Part model, mm, in its own coordinate system. Round coordinates to 2 decimals unless told otherwise and drop trailing zeros. Loops run counter-clockwise (first coordinate to the right, second up) from the corner with the lowest first, then second, coordinate; pieces in that order, holes last.
(1) Flat gauge pin, fed straight in: pin 1 (5 mm diameter, centred on x = 190, z = 155, fed in from +Y). Where does the tip first touch, or does it go through?
(2) Probe probe 1 along X at (y, z) = (-5.75, 204.5); probe 2 along X at (y, z) = (-4, 337.4); probe 3 along X at (y, z) = (-3.75, 125). List the from-to ranges inside material, lowest first.
(3) Cut at B-B on z = 61. List the corners of the cut face in (x, y), then the cut area to 3 significant figures.
(4) Cut at A-A on z = 125. List the corners of the cut face in (x, y), then the cut area to 3 significant figures.
(5) Cut at C-C on y = -8.25. Count the separate pieces of the cut face and the enclosed holes in it, then the cut area to 3 significant figures.
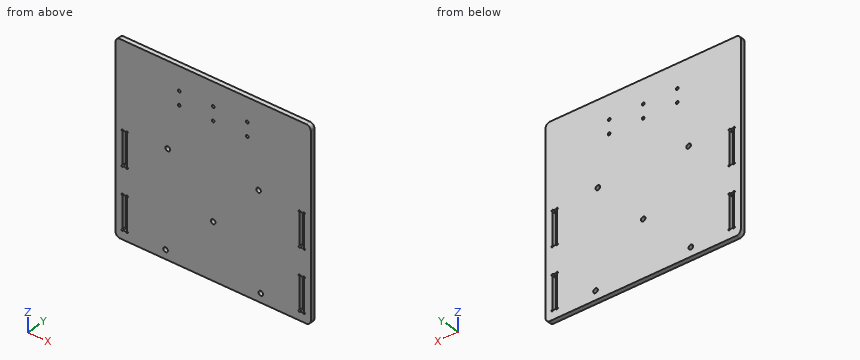
from build123d import *

# Parameters (mm, degrees)
F0_R     = 5.1
F0_R_2   = 3
F1_DEPTH = 10
F2_R     = 10


with BuildPart() as f1:
    # F0 (on Front) → F1 (new body)
    with BuildSketch(Plane.XZ):
        Polygon((-215, 0), (0, 0), (215, 0), (215, 420), (0, 420), (-215, 420), align=None)
        with BuildLine():
            ThreePointArc((-198, 20), (-201.414214, 18.585786), (-200, 22))
            Line((-200, 22), (-200, 93))
            ThreePointArc((-200, 93), (-201.414214, 96.414214), (-198, 95))
            Line((-198, 95), (-192, 95))
            ThreePointArc((-192, 95), (-188.585786, 96.414214), (-190, 93))
            Line((-190, 93), (-190, 22))
            ThreePointArc((-190, 22), (-188.585786, 18.585786), (-192, 20))
            Line((-192, 20), (-198, 20))
        make_face(mode=Mode.SUBTRACT)
        with Locations((-105, 20)):
            Circle(F0_R, mode=Mode.SUBTRACT)
        with BuildLine():
            Line((-192, 155), (-198, 155))
            ThreePointArc((-198, 155), (-201.414214, 153.585786), (-200, 157))
            Line((-200, 157), (-200, 228))
            ThreePointArc((-200, 228), (-201.414214, 231.414214), (-198, 230))
            Line((-198, 230), (-192, 230))
            ThreePointArc((-192, 230), (-188.585786, 231.414214), (-190, 228))
            Line((-190, 228), (-190, 157))
            ThreePointArc((-190, 157), (-188.585786, 153.585786), (-192, 155))
        make_face(mode=Mode.SUBTRACT)
        with Locations((105, 20)):
            Circle(F0_R, mode=Mode.SUBTRACT)
        with BuildLine():
            ThreePointArc((190, 93), (188.585786, 96.414214), (192, 95))
            Line((192, 95), (198, 95))
            ThreePointArc((198, 95), (201.414214, 96.414214), (200, 93))
            Line((200, 93), (200, 22))
            ThreePointArc((200, 22), (201.414214, 18.585786), (198, 20))
            Line((198, 20), (192, 20))
            ThreePointArc((192, 20), (188.585786, 18.585786), (190, 22))
            Line((190, 22), (190, 93))
        make_face(mode=Mode.SUBTRACT)
        with BuildLine():
            ThreePointArc((0, 119.9), (-5.1, 125), (0, 130.1))
            ThreePointArc((0, 130.1), (5.1, 125), (0, 119.9))
        make_face(mode=Mode.SUBTRACT)
        with BuildLine():
            Line((198, 155), (192, 155))
            ThreePointArc((192, 155), (188.585786, 153.585786), (190, 157))
            Line((190, 157), (190, 228))
            ThreePointArc((190, 228), (188.585786, 231.414214), (192, 230))
            Line((192, 230), (198, 230))
            ThreePointArc((198, 230), (201.414214, 231.414214), (200, 228))
            Line((200, 228), (200, 157))
            ThreePointArc((200, 157), (201.414214, 153.585786), (198, 155))
        make_face(mode=Mode.SUBTRACT)
        with Locations((-100, 234.8)):
            Circle(F0_R, mode=Mode.SUBTRACT)
        with Locations((-75, 337.4)):
            Circle(F0_R_2, mode=Mode.SUBTRACT)
        with Locations((-75, 367.4)):
            Circle(F0_R_2, mode=Mode.SUBTRACT)
        with Locations((100, 234.8)):
            Circle(F0_R, mode=Mode.SUBTRACT)
        with BuildLine():
            ThreePointArc((0, 340.4), (3, 337.4), (0, 334.4))
            ThreePointArc((0, 334.4), (-3, 337.4), (0, 340.4))
        make_face(mode=Mode.SUBTRACT)
        with BuildLine():
            ThreePointArc((0, 364.4), (-3, 367.4), (0, 370.4))
            ThreePointArc((0, 370.4), (3, 367.4), (0, 364.4))
        make_face(mode=Mode.SUBTRACT)
        with Locations((75, 337.4)):
            Circle(F0_R_2, mode=Mode.SUBTRACT)
        with Locations((75, 367.4)):
            Circle(F0_R_2, mode=Mode.SUBTRACT)
    extrude(amount=F1_DEPTH)

    # F2
    f2_edges = [f1.edges().sort_by_distance(p)[0] for p in [
        (215, -5, 0),
        (215, -5, 420),
        (-215, -5, 420),
        (-215, -5, 0),
    ]]
    fillet(f2_edges, radius=F2_R)


solid = f1.part
Final values:
1. pin 1: stops at y = 0
2. probe 1: x = -215 to -200, -190 to 190, 200 to 215
2. probe 2: x = -215 to -78, -72 to -3, 3 to 72, 78 to 215
2. probe 3: x = -215 to -5.1, 5.1 to 215
3. outline: (-215, -10) - (-200, -10) - (-200, 0) - (-215, 0) - close; (-190, -10) - (190, -10) - (190, 0) - (-190, 0) - close; (200, -10) - (215, -10) - (215, 0) - (200, 0) - close
3. area: 4,100 mm2
4. outline: (-215, -10) - (-5.1, -10) - (-5.1, 0) - (-215, 0) - close; (5.1, -10) - (215, -10) - (215, 0) - (5.1, 0) - close
4. area: 4,200 mm2
5. separate pieces: 1
5. enclosed holes: 15
5. area: 177,000 mm2
